Geometry: see drawing. Coordinates: mm, zero at the bounding-box minimum. Give positions to 0.01 mm unless a question says otherwise; leave off trailing zeros. Write each loop counter-clockwise with the first axis right and the second up, starting at its lowest first coordinate (ties: lowest second). Pieces come first, ordered by that corner, then holes. Notation, with made-up numbers: (-25.75, -34.75) -> (8.25, -34.75) arc R21 cw to (8.25, -18.75) -> close; hole circle Ø1 at (81, 80). An arc over 180 degrees is marked (long way). Answer as a JSON object with one key per item and string values. Group by question number.
Item 1: Section query A-A on z = 47.5. Return the cut outline in (x, y).
Item 2: Section query C-C on z = 40. Return the cut outline in (x, y).
Item 3: Section query B-B on y = 1.65. Give the number of separate pieces and of enclosed holes in the cut face, plus the area to 3 significant figures.
Item 4: Section query D-D on x = 3. Return the cut outline in (y, z).
Item 5: First-contact query: pin 1 Ø1.2 at (x, z) = (47, 10) entering from +Y. Flat tip, straight axial feed; report the tip coordinate or a pass-through.
Item 6: Ray query, probe 1 along X at (y, z) = (1.5, 47.5); probe 2 along X at (y, z) = (0.65, 10); probe 3 along Z at (x, y) = (2.5, 1.3). Return the intervals inside material, ascending. Write a range as from..to.
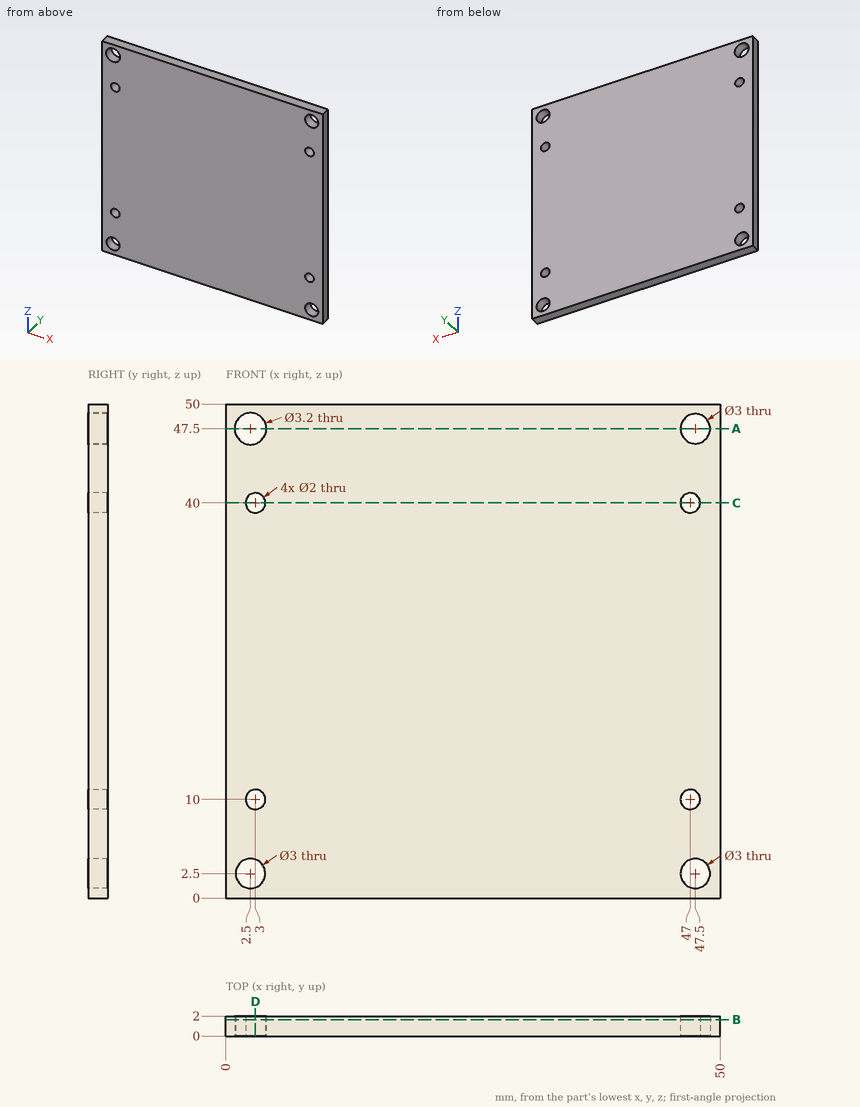
Worked answers:
{
 "1": {"outline": "(0, 0) -> (0.9, 0) -> (0.9, 2) -> (0, 2) -> close; (4.1, 0) -> (46, 0) -> (46, 2) -> (4.1, 2) -> close; (49, 0) -> (50, 0) -> (50, 2) -> (49, 2) -> close"},
 "2": {"outline": "(0, 0) -> (2, 0) -> (2, 2) -> (0, 2) -> close; (4, 0) -> (46, 0) -> (46, 2) -> (4, 2) -> close; (48, 0) -> (50, 0) -> (50, 2) -> (48, 2) -> close"},
 "3": {"separate pieces": "1", "enclosed holes": "8", "area": "2,460 mm^2"},
 "4": {"outline": "(0, 0) -> (2, 0) -> (2, 1.09) -> (0, 1.09) -> close; (0, 3.91) -> (2, 3.91) -> (2, 9) -> (0, 9) -> close; (0, 11) -> (2, 11) -> (2, 39) -> (0, 39) -> close; (0, 41) -> (2, 41) -> (2, 45.98) -> (0, 45.98) -> close; (0, 49.02) -> (2, 49.02) -> (2, 50) -> (0, 50) -> close"},
 "5": {"pin 1": "through"},
 "6": {"probe 1": "0..0.9, 4.1..46, 49..50", "probe 2": "0..2, 4..46, 48..50", "probe 3": "0..1, 4..9.13, 10.87..39.13, 40.87..45.9, 49.1..50"}
}
